Could you check a few things on this drawing? It's one solid part, dimensions in mm from its lowest x, y, z. A direction names the side the tool comes from. Round coordinates to 2 decimals unless told otherwise and drop trailing zeros. Write each loop counter-clockwise with the first axis right and the second up, starting at its lowest first coordinate (ties: lowest second). Pieces come first, ordered by that corner, then holes. Notation, with made-up numbers: (-5, -20.5) -> (43, -20.5) arc R11 cw to (43, -3.5) -> close; hole circle Ø3 at (-13.75, 13.5). An arc over 180 degrees is marked (long way). Answer as CSV lines item,"result".
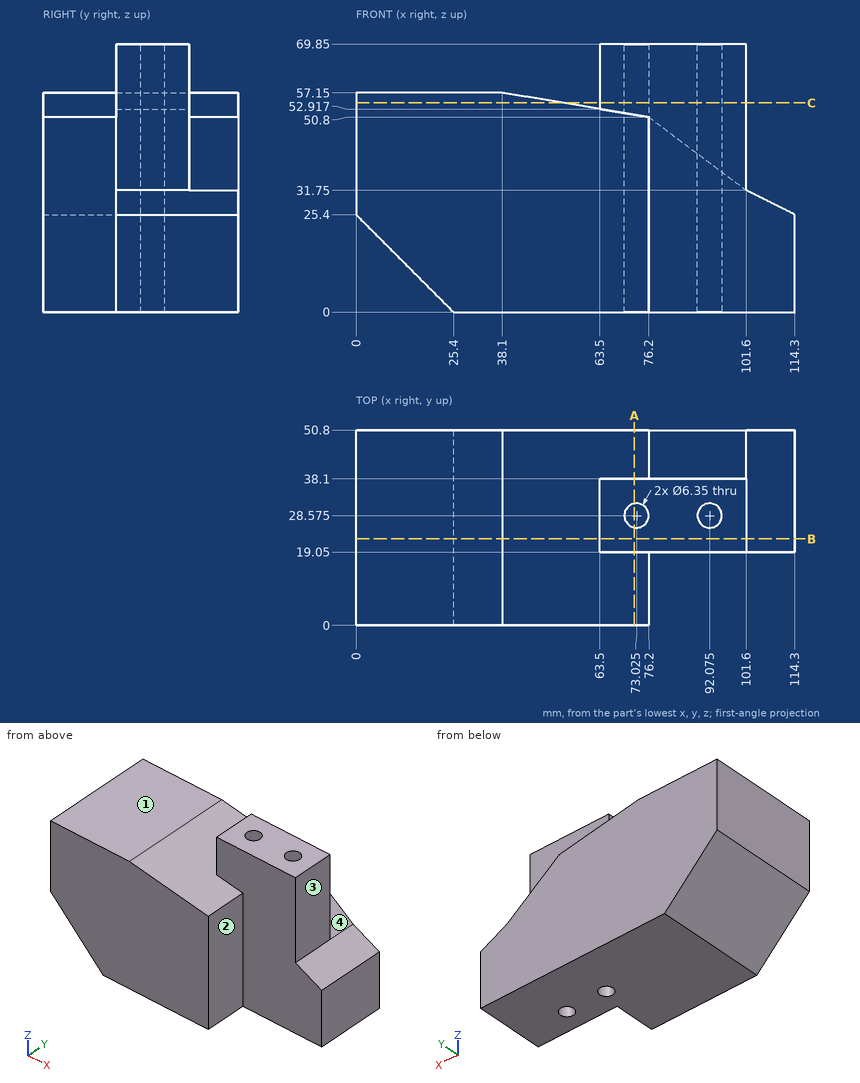
1. If I drill on line 1 (Z direction, x = 37, y = 19); line 2 (X direction, y = 22.5, z = 50); line 3 (Y direction, x = 92, z = 8), over which ranges is the centre line in solid material (lowest first)?
Numbers:
line 1,"z = 0 to 57.15"
line 2,"x = 0 to 101.6"
line 3,"y = 19.05 to 25.4, 31.75 to 50.8"
2. On a 3-axis mill with a long thin cutter (end or side, diameter ignored), from which of +Z, -Z, +X, -X, +Y, -Y can I reach the whole of each face in a straight line? I mean the marked faces 1, 2, 3 and 4. Say none if no direction works.
Numbers:
face 1,"+Z, -X, +Y, -Y"
face 2,"+Z, -Z, +X, -Y"
face 3,"+Z, +X, +Y, -Y"
face 4,"+Z, +X, +Y"
3. For pin 1 Ø5.5 at (x, y) = (73.025, 28.575) entering from -Z; pin 2 Ø9.5 at (y, z) = (12, 33) entering from +X; pin 3 Ø2 at (x, z) = (97.5, 57.5) entering from -Y; pin 4 Ø9.5 at (y, z) = (33, 42) entering from +X, each with a flat end and sliding along its axis, tell me the tip position at first contact or that it passes through.
Numbers:
pin 1,"passes through"
pin 2,"stops at x = 76.2"
pin 3,"stops at y = 19.05"
pin 4,"stops at x = 101.6"
4. Suppose I cut it at C-C on z = 54.5. Count the separate pieces of the cut face and the enclosed holes in it, and give its area (3 significant figures).
Numbers:
separate pieces,"2"
enclosed holes,"2"
area,"3,410 mm^2"
5. Suppose I cut it at B-B on y = 22.5. Please give me the cut outline in (x, z), and give its area (3 significant figures).
Numbers:
outline,"(0, 25.4) -> (25.4, 0) -> (114.3, 0) -> (114.3, 25.4) -> (101.6, 31.75) -> (101.6, 69.85) -> (63.5, 69.85) -> (63.5, 52.92) -> (38.1, 57.15) -> (0, 57.15) -> close"
area,"6,280 mm^2"
6. Suppose I cut it at A-A on x = 72.5. Please give me the cut outline in (y, z).
Numbers:
outline,"(0, 0) -> (25.44, 0) -> (25.44, 69.85) -> (19.05, 69.85) -> (19.05, 51.42) -> (0, 51.42) -> close; (31.71, 0) -> (50.8, 0) -> (50.8, 51.42) -> (38.1, 51.42) -> (38.1, 69.85) -> (31.71, 69.85) -> close"
